Geometry: final body of the model. Coordinates: model frame, mm. A direction names the side the tool comes from. Give positions to 0.01 mm unless a question says otherwise; leave off trailing zeros. Loops run counter-clockwise (first coordinate to the right, second up) from the corner with the lowest first, then second, coordinate; pieces in that order, holes last.
1. Section C-C, the plane z = 7.5. Output: boundary loops of the cut face in (x, y).
2. Section A-A, the plane y = 0. Output: boundary loops of the cut face in (x, z), then the cut area to 3 significant figures.
3. Material intervals for line 1 along Y through (x, z) = (10, 6); line 2 along Y through (x, z) = (-20, 4.5); line 3 along Y through (x, z) = (14, 4), sorted ascending.
4. Section D-D, the plane x = -11. Output: boundary loops of the cut face in (y, z).
5. Draft query along X for faces 1 (the face through (12.5, 0, 4.9)), 2 (the face through (-25, 0, 5)), 3 (the face through (15.19, -25.87, 4.93)). Return one class per face: +X half, -X half, draft (parallel to the pull), parting line (faces both ways), or undercut.
6. First-contact query: P1, Ø1.5, axis at x = -5, z = 4, coming from the +Y side; P2, Ø3, axis at y = -17.5, z = 9, coming from the -X side; P3, Ø6, axis at x = -20, y = 0, coming from the +Z side; P4, Ø1, axis at x = -11, z = 1, coming from the -Y side. Flat tips, straight axial feed; report the tip coordinate or a pass-through.
7. Section B-B, the plane x = 10. Output: boundary loops of the cut face in (y, z), then the cut area to 3 significant figures.
8. Access query for faces 4 (the face through (-14, -10, 5)), 5 (the face through (1, 0, 10)), 6 (the face through (15.579, 6.984, 4.93)), 7 (the face through (-14, 10, 5)). Directions: +Z, -Z, +X, -X, +Y, -Y. A direction counts if a zero-diameter tool reaches every point of the face in a straight line with its end or side. Return the directions, or none.
from build123d import *

# Parameters (mm, degrees)
CROQUIS1_R              = 5
SALIENTE_EXTRUIR1_DEPTH = 10


with BuildPart() as part:
    # Croquis1 → Saliente-Extruir1 (new body)
    with BuildSketch(Plane.XY):
        with BuildLine():
            Line((-20, 10), (-7.5, 10))
            ThreePointArc((-7.5, 10), (-6.25, 10.825317547), (-4.910254038, 11.495190528))
            Line((-4.910254038, 11.495190528), (1.339745962, 22.320508076))
            ThreePointArc((1.339745962, 22.320508076), (15, 25.980762114), (18.660254038, 12.320508076))
            Line((18.660254038, 12.320508076), (12.410254038, 1.495190528))
            ThreePointArc((12.410254038, 1.495190528), (12.499999989, 0), (12.410254038, -1.495190528))
            Line((12.410254038, -1.495190528), (18.660254038, -12.320508076))
            ThreePointArc((18.660254038, -12.320508076), (15, -25.980762114), (1.339745962, -22.320508076))
            Line((1.339745962, -22.320508076), (-4.910254038, -11.495190528))
            ThreePointArc((-4.910254038, -11.495190528), (-6.25, -10.825317547), (-7.5, -10))
            Line((-7.5, -10), (-20, -10))
            ThreePointArc((-20, -10), (-30, 0), (-20, 10))
        make_face()
        with Locations((-20, 0)):
            Circle(CROQUIS1_R, mode=Mode.SUBTRACT)
        with Locations((10, 17.320508076)):
            Circle(CROQUIS1_R, mode=Mode.SUBTRACT)
        with Locations((10, -17.320508076)):
            Circle(CROQUIS1_R, mode=Mode.SUBTRACT)
    extrude(amount=SALIENTE_EXTRUIR1_DEPTH)


solid = part.part
Answers below:
1. outline: (-20, -10) - (-7.5, -10) arc R12.5 ccw to (-4.91, -11.5) - (1.34, -22.32) arc R10 ccw to (18.66, -12.32) - (12.41, -1.5) arc R12.5 ccw to (12.41, 1.5) - (18.66, 12.32) arc R10 ccw to (1.34, 22.32) - (-4.91, 11.5) arc R12.5 ccw to (-7.5, 10) - (-20, 10) arc R10 ccw to start; hole circle Ø10 at (-20, 0); hole circle Ø10 at (10, -17.32); hole circle Ø10 at (10, 17.32)
2. outline: (-30, 0) - (-25, 0) - (-25, 10) - (-30, 10) - close; (-15, 0) - (12.5, 0) - (12.5, 10) - (-15, 10) - close
2. area: 325 mm2
3. line 1: y = -27.32 to -22.32, -12.32 to 12.32, 22.32 to 27.32
3. line 2: y = -10 to -5, 5 to 10
3. line 3: y = -26.49 to -20.32, -14.32 to -4.25, 4.25 to 14.32, 20.32 to 26.49
4. outline: (-10, 0) - (10, 0) - (10, 10) - (-10, 10) - close
5. face 1: +X half
5. face 2: undercut
5. face 3: parting line
6. P1: stops at y = 12.64
6. P2: stops at x = -2.31
6. P3: passes through
6. P4: stops at y = -10
7. outline: (-27.32, 0) - (-22.32, 0) - (-22.32, 10) - (-27.32, 10) - close; (-12.32, 0) - (12.32, 0) - (12.32, 10) - (-12.32, 10) - close; (22.32, 0) - (27.32, 0) - (27.32, 10) - (22.32, 10) - close
7. area: 346 mm2
8. face 4: +Z, -Z, -X, -Y
8. face 5: +Z, +X, -X, +Y, -Y
8. face 6: +Z, -Z, +X
8. face 7: +Z, -Z, -X, +Y
